from build123d import *

# Parameters (mm, degrees)
F0_R      = 30.528215
F1_DEPTH  = 86.868
F2_R      = 19.622728
F1_FACE_R = 10.905488
F3_DEPTH  = 42.418


with BuildPart() as f1:
    # F0 (on Front) → F1 (new body)
    with BuildSketch(Plane.XZ):
        Circle(F0_R)
    extrude(amount=-F1_DEPTH)

    # F2
    f2_edges = [f1.edges().sort_by_distance(p)[0] for p in [
        (-30.528215, 86.868, 0),
    ]]
    fillet(f2_edges, radius=F2_R)

    # F1_face (on face) → F3 (join)
    with BuildSketch(Plane(origin=(0, 86.868, 0), x_dir=(1, 0, 0), z_dir=(0, 1, 0))):
        Circle(F1_FACE_R)
    extrude(amount=F3_DEPTH)


solid = f1.part
For this review, take the finished solid that the model builds, in its own axes (mm). A direction names the side the tool comes from. Give positions to 0.01 mm unless a question says otherwise; leave off trailing zeros. Loops run counter-clockwise (first coordinate to the right, second up) from the corner with the lowest first, then second, coordinate; pieces in that order, holes last. Notation, with made-up numbers: M 36.5,-35.75 L 49.5,-35.75 A17 cw 49.5,-21.75 Z; hole C 12,71.5 d7. An arc over 180 degrees is marked long. Put each result on its own line as item: value. Start each with the question number.
(1) Add section B-B, the plane y = 21. Write out the cut boundary in (x, z), then the cut area to 3 significant figures.
(2) Add section A-A, the plane y = 100.5. Write out the cut boundary in (x, z), then the cut area to 3 significant figures.
(3) Wall thickness on L1, parallel to Z at x = -8, y = 102; L2, parallel to X at y = 40, z = -5.5; L3, parallel to X at y = 47.5, z = 5: over which ranges is each line inside the solid? List them lowest first.
(4) Machinability: for faces 1 (the cylindrical face through (10.4, 107.78, -3.28)), 2 (the flat face through (0, 0, 0)), which of the approach directions +Z, -Z, +X, -X, +Y, -Y give a long, thin tool a straight path to every point of the face, cutting with its end or side? Answer none if there is none.
(5) For pin 1 (5 mm diameter, centred on y = 99, z = -1.5, fed in from -X); pin 2 (8 mm diameter, centred on x = -23.5, y = 70.5, fed in from -Z); pin 3 (1.5 mm diameter, centred on x = 7.5, z = -21, fed in from +Y), all flat-tipped, find the tip position at first contact; note any pin that passes through.
Result:
1. outline: C 0,0 d61.06
1. area: 2,930 mm^2
2. outline: C 0,0 d21.81
2. area: 374 mm^2
3. L1: z = -7.41 to 7.41
3. L2: x = -30.03 to 30.03
3. L3: x = -30.12 to 30.12
4. face 1: +Y
4. face 2: +Z, -Z, +X, -X, -Y
5. pin 1: stops at x = -10.91
5. pin 2: stops at z = -23.22
5. pin 3: stops at y = 83.73
